Check sheet for the modelled part. Datum: model origin and axes. Units: mm. A direction names the side the tool comes from. Coordinates: 2 decimals unless noted, no trailing zeros. Order: outer loops, then holes, each group sorted by start corner. A loop starts at its lowest first (then second) coordinate and runs counter-clockwise, first axis right, second up.
from build123d import *

# Parameters (mm, degrees)
SKETCH007_W     = 500
SKETCH007_H     = 400
SKETCH007_W_2   = 447
SKETCH007_H_2   = 347
PAD002_DEPTH    = 47
PAD003_DEPTH    = 380
PAD003_FACE11_W = 7.3
PAD003_FACE11_H = 380
POCKET002_DEPTH = 5


with BuildPart() as part:
    # Sketch007 → Pad002 (new body)
    with BuildSketch(Plane.XY):
        Rectangle(SKETCH007_W, SKETCH007_H)
        Rectangle(SKETCH007_W_2, SKETCH007_H_2, mode=Mode.SUBTRACT)
    extrude(amount=PAD002_DEPTH)

    # Sketch008 (on Face5 of Pad002) → Pad003 (join)
    with BuildSketch(Plane.YZ.offset(-223.5)):
        Polygon((183.1, 42), (183.1, 47), (190.4, 47), (190.4, 42), (189.4, 42), (189.4, 46), (184.1, 46), (184.1, 42), align=None)
    extrude(amount=PAD003_DEPTH)

    # Pad003 Face11 → Pocket002 (cut)
    with BuildSketch(Plane(origin=(-33.5, 186.75, 47), x_dir=(0, 1, 0), z_dir=(0, 0, 1))):
        Rectangle(PAD003_FACE11_W, PAD003_FACE11_H)
    extrude(amount=-POCKET002_DEPTH, mode=Mode.SUBTRACT)


solid = part.part
(1) Thickness scan on probe 1 along Y at (x, z) = (9.5, 5.5); probe 2 along X at (y, z) = (-162, 37). Record the ranges inside material, lowest first.
Filled in:
probe 1: y = -200 to -173.5, 173.5 to 200
probe 2: x = -250 to -223.5, 223.5 to 250
(2) Tool access check on faces 4 (the flat face through (-20, -177, 47)), 5 (the flat face through (-3, -173.5, 23)). Record the directions out of +Z, -Z, +X, -X, +Y, -Y that give a thin tool (end or side, any length) a straight path to the whole face; none if there is none.
Filled in:
face 4: +Z, +X, -X, +Y, -Y
face 5: +Z, -Z
(3) Release check for a two-part mould opening along X. For faces 1 (the flat face through (-223.5, -2, 23)), 2 (the flat face through (-250, -3, 23)), 3 (the flat face through (-3, 200, 23)) record: +X half, -X half, draft (parallel to the pull), parting line (faces both ways), or undercut.
Filled in:
face 1: undercut
face 2: -X half
face 3: draft
(4) Cross-section at A-A (y = 85). Enter the section's corners in (x, z).
Filled in:
outline: (-250, 0) - (-223.5, 0) - (-223.5, 47) - (-250, 47) - close; (223.5, 0) - (250, 0) - (250, 47) - (223.5, 47) - close
(5) Cross-section at C-C (x = -209). Enter the section's corners in (y, z), and give its area (3 significant figures).
Filled in:
outline: (-200, 0) - (-173.5, 0) - (-173.5, 47) - (-200, 47) - close; (173.5, 0) - (200, 0) - (200, 47) - (190.4, 47) - (190.4, 42) - (183.1, 42) - (183.1, 47) - (173.5, 47) - close
area: 2,450 mm2
(6) Cross-section at B-B (z = 9). Enter the section's corners in (x, y).
Filled in:
outline: (-250, -200) - (250, -200) - (250, 200) - (-250, 200) - close; hole (-223.5, -173.5) - (223.5, -173.5) - (223.5, 173.5) - (-223.5, 173.5) - close
